from build123d import *

# Parameters (mm, degrees)
SKETCH_1_R               = 10
SKETCH_1_R_2             = 8.75
EXTRUDE_1_DEPTH          = 115
CUT_EXTRUDE_1_DEPTH      = 116.866302263
CUT_EXTRUDE_1_DEPTH_BACK = 116.866302263
SKETCH_2_R               = 3


with BuildPart() as part:
    # 草图1 → 凸台-拉伸1 (new body)
    with BuildSketch(Plane(origin=(0, 0, 0), x_dir=(0, 0, -1), z_dir=(1, 0, 0))):
        Circle(SKETCH_1_R)
        Circle(SKETCH_1_R_2, mode=Mode.SUBTRACT)
    extrude(amount=EXTRUDE_1_DEPTH)

    # 草图2 → 切除-拉伸1 (cut, two sides: drawn at the far end of the back side and taken through both)
    with BuildSketch(Plane(origin=(0, 0, 0), x_dir=(1, 0, 0), z_dir=(0, 1, 0)).offset(-CUT_EXTRUDE_1_DEPTH_BACK)):
        with Locations(Location((20, 0, 0), (0, 0, 270))):
            Circle(SKETCH_2_R)
        with Locations(Location((95, 0, 0), (0, 0, 270))):
            Circle(SKETCH_2_R)
    extrude(amount=CUT_EXTRUDE_1_DEPTH + CUT_EXTRUDE_1_DEPTH_BACK, mode=Mode.SUBTRACT)


solid = part.part
Geometry: final body of the model. Coordinates: model frame, mm. Give positions to 0.01 mm unless a question says otherwise; leave off trailing zeros. Loops run counter-clockwise (first coordinate to the right, second up) from the corner with the lowest first, then second, coordinate; pieces in that order, holes last. Notation, with made-up numbers: (-29.75, 69) - (3.25, 69) arc R9 ccw to (3.25, 73) - close; hole circle Ø10 at (22, 11.5). An arc over 180 degrees is marked (long way). Answer as CSV lines item,"result". Start each with the question number.
1. Section A-A, the plane y = 0. Return loops of the section in (x, z).
2. Section D-D, the plane z = 2. Return loops of the section in (x, y).
3. Draft query along X for faces 1 (the face through (56.695, -3.83, -9.237)), 2 (the face through (115, -9, 0)), 3 (the face through (95, 9, -3)), 4 (the face through (17.07, -9.13, -0.65)). Return one class per face: released by +X, released by -X, zero draft, split by the parting line, or undercut.
4. Section C-C, the plane x = 30. Return loops of the section in (y, z), plus the area to 3 significant figures.
5. Ray query, L1, parallel to X at y = -9.1, z = 0; L2, parallel to Y at x = 85.5, z = 0; L3, parallel to Z at x = 73, y = 5.5. Return the intervals inside material, ascending.
6. Section B-B, the plane z = -4.5. Return loops of the section in (x, y), plus the area to 3 significant figures.
7. Pin query (flat end, axial travel): P1, Ø2, axis at x = 87, z = 3, coming from the -Y side; P2, Ø9.5, axis at x = 20, z = 0, coming from the +Y side; P3, Ø4, axis at x = 33, z = -3.5, coming from the -Y side; P4, Ø6, axis at x = 44.5, y = 6, coming from the -Z side. Return the tip coordinate at first contact, or that it passes through.
Answers:
1,outline,"(0, -10) - (115, -10) - (115, -8.75) - (0, -8.75) - close; (0, 8.75) - (115, 8.75) - (115, 10) - (0, 10) - close"
2,outline,"(0, -9.8) - (17.76, -9.8) - (17.76, -8.52) - (0, -8.52) - close; (0, 8.52) - (17.76, 8.52) - (17.76, 9.8) - (0, 9.8) - close; (22.24, -9.8) - (92.76, -9.8) - (92.76, -8.52) - (22.24, -8.52) - close; (22.24, 8.52) - (92.76, 8.52) - (92.76, 9.8) - (22.24, 9.8) - close; (97.24, -9.8) - (115, -9.8) - (115, -8.52) - (97.24, -8.52) - close; (97.24, 8.52) - (115, 8.52) - (115, 9.8) - (97.24, 9.8) - close"
3,face 1,"zero draft"
3,face 2,"released by +X"
3,face 3,"undercut"
3,face 4,"undercut"
4,outline,"circle Ø20 at (0, 0); hole circle Ø17.5 at (0, 0)"
4,area,"73.6 mm2"
5,L1,"x = 0 to 17, 23 to 92, 98 to 115"
5,L2,"y = -10 to -8.75, 8.75 to 10"
5,L3,"z = -8.35 to -6.81, 6.81 to 8.35"
6,outline,"(0, -8.93) - (115, -8.93) - (115, -7.5) - (0, -7.5) - close; (0, 7.5) - (115, 7.5) - (115, 8.93) - (0, 8.93) - close"
6,area,"328 mm2"
7,P1,"stops at y = -9.8"
7,P2,"stops at y = 10"
7,P3,"stops at y = -9.89"
7,P4,"stops at z = -9.54"
